Geometry check sheet. Reference: the model listing, model coordinates, mm. A direction names the side the tool comes from. Give positions to 0.01 mm unless a question says otherwise; leave off trailing zeros. Loops run counter-clockwise (first coordinate to the right, second up) from the corner with the lowest first, then second, coordinate; pieces in that order, holes last. Notation, with made-up numbers: (72, 47) -> (79, 47) arc R34 ccw to (79, 78) -> close; hole circle Ø5 at (-4, -27.5). An arc over 180 degrees is marked (long way). Write item = value, one per line. Start each with the question number.
```python
from build123d import *

# Parameters (mm, degrees)
SKETCH_1_R          = 1
EXTRUDE_1_DEPTH     = 30
CUT_EXTRUDE_1_REACH = 81.318
SKETCH_2_W          = 6
SKETCH_2_H          = 12


with BuildPart() as part:
    # Эскиз1 → Бобышка-Вытянуть1 (new body)
    with BuildSketch(Plane.XY):
        with BuildLine():
            Line((-15, 20), (-12.857189373, 20))
            Line((-12.857189373, 20), (-12.857189373, 6))
            Line((-12.857189373, 6), (-15, 6))
            ThreePointArc((-15, 6), (-18, 3), (-15, 0))
            Line((-15, 0), (0, 0))
            Line((0, 0), (0, 55.160876672))
            Line((0, 55.160876672), (0, 71.184974766))
            Line((0, 71.184974766), (-12.857189373, 71.184974766))
            Line((-12.857189373, 71.184974766), (-12.857189373, 26))
            Line((-12.857189373, 26), (-15, 26))
            ThreePointArc((-15, 26), (-18, 23), (-15, 20))
        make_face()
        with Locations((-15, 23)):
            Circle(SKETCH_1_R, mode=Mode.SUBTRACT)
        with Locations((-15, 3)):
            Circle(SKETCH_1_R, mode=Mode.SUBTRACT)
    extrude_1 = extrude(amount=-EXTRUDE_1_DEPTH)

    # Вырез-Вытянуть1: up to this face of the body (flat: up to its plane)
    cut_extrude_1_end = Plane(part.part.faces().sort_by_distance((-13.928594687, 26, -15))[0])
    # Эскиз2 → Вырез-Вытянуть1 (cut, up to the picked face)
    with BuildSketch(Plane(origin=(0, 0, 0), x_dir=(1, 0, 0), z_dir=(0, 1, 0)), mode=Mode.PRIVATE) as cut_extrude_1_sk1:
        with Locations((-15, 15)):
            Rectangle(SKETCH_2_W, SKETCH_2_H)
    cut_extrude_1_tool1 = split(extrude(cut_extrude_1_sk1.sketch, amount=CUT_EXTRUDE_1_REACH, mode=Mode.PRIVATE), bisect_by=cut_extrude_1_end, keep=Keep.BOTH, mode=Mode.PRIVATE)
    cut_extrude_1 = cut_extrude_1_tool1.solids().sort_by(Axis((-15, 0, -15), (0, 1, 0)))[0]
    add(cut_extrude_1, mode=Mode.SUBTRACT)

    # Зеркальное отражение1: Бобышка-Вытянуть1, Вырез-Вытянуть1 across plane
    add(extrude_1.mirror(Plane(origin=(0, 71.184974766, -30), x_dir=(0, 0, 1), z_dir=(1, 0, 0))))
    add(cut_extrude_1.mirror(Plane(origin=(0, 71.184974766, -30), x_dir=(0, 0, 1), z_dir=(1, 0, 0))), mode=Mode.SUBTRACT)


solid = part.part
```
1) Section check C-C (z = -7.75). Enter the section's corners in (x, y).
2) Section check B-B (y = 23). Enter the section's corners in (x, z), plus the area to 3 significant figures.
3) Depth check by flat-ended pin: pin 1 Ø1.2 at (x, y) = (-15, 3) entering from -Z (3 decimals); pin 2 Ø1.7 at (x, z) = (14, -23.5) entering from +Y; pin 3 Ø7 at (y, z) = (16, -6.5) entering from +X; pin 4 Ø3 at (y, z) = (17.5, -16.5) entering from +X. Enter the tip coordinate at first touch or a pass-through.
4) Thickness scan on line 1 (Y direction, x = 15, z = -23); line 2 (Z direction, x = 13, y = 4.5); line 3 (X direction, y = 64.5, z = -8.75). Record the ranges inside material, lowest first.
5) Section check A-A (z = -18.75). Enter the section's corners in (x, y).
6) Tool access check on faces 1 (the flat face through (14, 20, -4)), 2 (the flat face through (-12.857, 49, -15)), 3 (the flat face through (-12.4, 12.8, -9)), 4 (the flat face through (14, 26, -4)). Record the directions out of +Z, -Z, +X, -X, +Y, -Y that give a thin tool (end or side, any length) a straight path to the whole face; none if there is none.
7) Draft check along Y on faces 5 (the flat face through (12.857, 13, -4)), 6 (the flat face through (12, 13, -15)), 7 (the flat face through (0, 71.185, -15)), 8 (the flat face through (14, 6, -25)). Enter one of: released by +Y, released by -Y, zero draft, split by the parting line, or undercut.
8) Section check D-D (y = 37). Enter the section's corners in (x, z), plus the area to 3 significant figures.
Check result:
q1.outline = (-15, 0) -> (15, 0) arc R3 ccw to (15, 6) -> (12.86, 6) -> (12.86, 20) -> (15, 20) arc R3 ccw to (15, 26) -> (12.86, 26) -> (12.86, 71.18) -> (-12.86, 71.18) -> (-12.86, 26) -> (-15, 26) arc R3 ccw to (-15, 20) -> (-12.86, 20) -> (-12.86, 6) -> (-15, 6) arc R3 ccw to start; hole circle Ø2 at (-15, 3); hole circle Ø2 at (-15, 23); hole circle Ø2 at (15, 3); hole circle Ø2 at (15, 23)
q2.outline = (-18, -30) -> (-16, -30) -> (-16, -21) -> (-18, -21) -> close; (-18, -9) -> (-16, -9) -> (-16, 0) -> (-18, 0) -> close; (-14, -30) -> (14, -30) -> (14, -21) -> (12, -21) -> (12, -9) -> (14, -9) -> (14, 0) -> (-14, 0) -> (-14, -9) -> (-12, -9) -> (-12, -21) -> (-14, -21) -> close; (16, -30) -> (18, -30) -> (18, -21) -> (16, -21) -> close; (16, -9) -> (18, -9) -> (18, 0) -> (16, 0) -> close
q2.area = 864 mm2
q3.pin_1 = through
q3.pin_2 = 26
q3.pin_3 = 12.86
q3.pin_4 = 12
q4.line_1 = 0 to 2, 4 to 6, 20 to 22, 24 to 26
q4.line_2 = -30 to -21, -9 to 0
q4.line_3 = -12.86 to 12.86
q5.outline = (-12.86, 26) -> (-12, 26) -> (-12, 0) -> (12, 0) -> (12, 26) -> (12.86, 26) -> (12.86, 71.18) -> (-12.86, 71.18) -> close
q6.face_1 = +Z, -Z, +X
q6.face_2 = +Z, -Z, -X, +Y
q6.face_3 = -X, -Y
q6.face_4 = +Z, -Z, +X, +Y
q7.face_5 = undercut
q7.face_6 = zero draft
q7.face_7 = released by +Y
q7.face_8 = undercut
q8.outline = (-12.86, -30) -> (12.86, -30) -> (12.86, 0) -> (-12.86, 0) -> close
q8.area = 771 mm2
